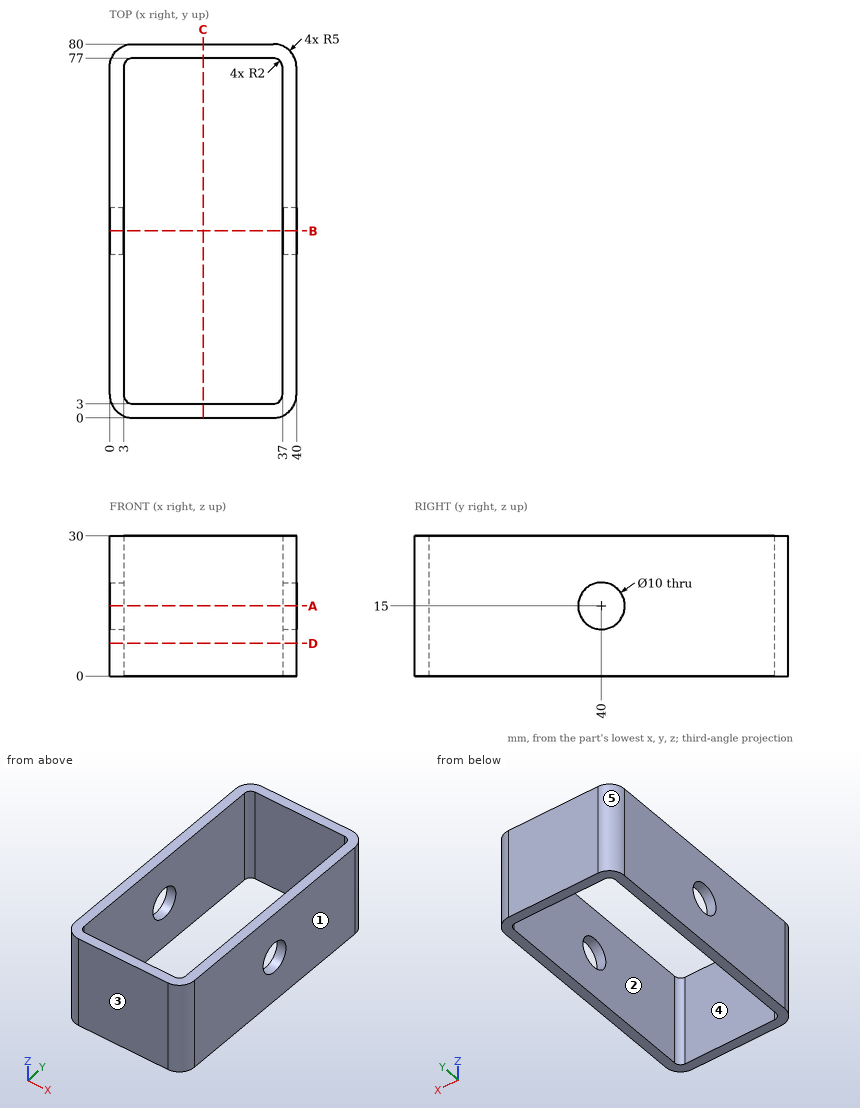
Can you work these out from the drawing? Everything is in mm from the part's minimum corner. A direction names the side the tool comes from. Coordinates: 2 decimals unless noted, no trailing zeros. Loops run counter-clockwise (first coordinate to the right, second up) from the corner with the lowest first, then second, coordinate; pieces in that order, holes last. Notation, with made-up numbers: (45.5, 33.25) -> (51.5, 33.25) arc R22 cw to (51.5, 72.25) -> close; hole circle Ø5 at (-14.5, 38). An arc over 180 degrees is marked (long way). Return JSON: item names as keys, results as strings.
1) If we section it at D-D, the plane z = 7: Write out the boundary of the cut face in (x, y).
Results below:
{"outline": "(0, 5) arc R5 ccw to (5, 0) -> (35, 0) arc R5 ccw to (40, 5) -> (40, 75) arc R5 ccw to (35, 80) -> (5, 80) arc R5 ccw to (0, 75) -> close; hole (3, 5) arc R2 ccw to (5, 3) -> (35, 3) arc R2 ccw to (37, 5) -> (37, 75) arc R2 ccw to (35, 77) -> (5, 77) arc R2 ccw to (3, 75) -> close"}
2) For the marked faces 1 and 2, which set-ups out of +Z, -Z, +X, -X, +Y, -Y let a thin tool reach every point of the face, with its end or its side?
Results below:
{"face 1": "+Z, -Z, +X, +Y, -Y", "face 2": "+Z, -Z"}
3) Thinking about a two-plate mould opening in Y: for the marked faces 3, 4 and 5, which applies, +Y half, -Y half, draft (parallel to the pull), parting line (faces both ways), or undercut?
Results below:
{"face 3": "-Y half", "face 4": "undercut", "face 5": "+Y half"}
4) I need wall thicknesses on line 1 (X direction, y = 38, z = 20.25); line 2 (Y direction, x = 5, z = 16.75); line 3 (Z direction, x = 2.4, y = 40). Which ranges of each line are inside material? Lowest first, please. Write a range as from..to.
Results below:
{"line 1": "0..3, 37..40", "line 2": "0..3, 77..80", "line 3": "0..10, 20..30"}
5) If we section it at A-A, the plane z = 15: Write out the boundary of the cut face in (x, y), then the cut area to 3 significant figures.
Results below:
{"outline": "(0, 5) arc R5 ccw to (5, 0) -> (35, 0) arc R5 ccw to (40, 5) -> (40, 35) -> (37, 35) -> (37, 5) arc R2 cw to (35, 3) -> (5, 3) arc R2 cw to (3, 5) -> (3, 35) -> (0, 35) -> close; (0, 45) -> (3, 45) -> (3, 75) arc R2 cw to (5, 77) -> (35, 77) arc R2 cw to (37, 75) -> (37, 45) -> (40, 45) -> (40, 75) arc R5 ccw to (35, 80) -> (5, 80) arc R5 ccw to (0, 75) -> close", "area": "606 mm²"}
6) If we section it at B-B, the plane y = 40: Write out the boundary of the cut face in (x, z).
Results below:
{"outline": "(0, 0) -> (3, 0) -> (3, 10) -> (0, 10) -> close; (0, 20) -> (3, 20) -> (3, 30) -> (0, 30) -> close; (37, 0) -> (40, 0) -> (40, 10) -> (37, 10) -> close; (37, 20) -> (40, 20) -> (40, 30) -> (37, 30) -> close"}
7) If we section it at C-C, the plane x = 20: Write out the boundary of the cut face in (y, z).
Results below:
{"outline": "(0, 0) -> (3, 0) -> (3, 30) -> (0, 30) -> close; (77, 0) -> (80, 0) -> (80, 30) -> (77, 30) -> close"}
